Here's how the part is built. I have some questions about the finished solid (model axes, mm). A direction names the side the tool comes from. Round coordinates to 2 decimals unless told otherwise and drop trailing zeros. Write each loop counter-clockwise with the first axis right and the second up, starting at its lowest first coordinate (ties: lowest second). Pieces come first, ordered by that corner, then holes. Notation, with made-up numbers: (-36.5, 71.25) - (-7.5, 71.25) arc R10 ccw to (-7.5, 85.25) - close; hole circle Ø6 at (67.25, -0.75). An arc over 180 degrees is marked (long way). Return JSON: item names as keys, results as strings. Group by question number.
Autodesk Inventor part; units mm, degrees
ref_plane "YZ Plane" through (0, 0, 0) normal (1, 0, 0) x (0, 1, 0)
ref_plane "XZ Plane" through (0, 0, 0) normal (0, 1, 0) x (-1, 0, 0)
ref_plane "XY Plane" through (0, 0, 0) normal (0, 0, 1) x (1, 0, 0)
sketch "Sketch1" plane through (0, 0, 0) normal (0, 0, 1) x (1, 0, 0)
  line L0 (0, 0) -> (111, 0)
  line L1 (111, 0) -> (111, 66)
  line L2 (111, 66) -> (0, 66)
  line L3 (0, 66) -> (0, 0)
  line L4 (2, 2) -> (109, 2)
  line L5 (109, 2) -> (109, 64)
  line L6 (109, 64) -> (2, 64)
  line L7 (2, 64) -> (2, 2)
  line L8 (2, 64) -> (107, 64)
  line L9 (107, 64) -> (107, 2)
  line L10 (107, 2) -> (2, 2)
  line L11 (2, 2) -> (2, 64)
  line L12 (2, 64) -> (0, 64)
  line L13 (0, 64) -> (0, 2)
  line L14 (0, 2) -> (2, 2)
  line L15 (2, 2) -> (2, 64)
  line L16 (2, 64) -> (107, 64)
  line L17 (107, 64) -> (107, 62)
  line L18 (107, 62) -> (2, 62)
  line L19 (2, 62) -> (2, 64)
  line L20 (2, 2) -> (107, 2)
  line L21 (107, 2) -> (107, 4)
  line L22 (107, 4) -> (2, 4)
  line L23 (2, 4) -> (2, 2)
  point P0 (2, 64)
  point P1 (2, 2)
  point P2 (107, 2)
  point P3 (2, 4)
  point P4 (2, 62)
  dimension "d0" = 111
  dimension "d1" = 66
  dimension "d2" = 107
  dimension "d3" = 2
  dimension "d4" = 2
  dimension "d5" = 62
  dimension "d6" = 105
  dimension "d8" = 0
  dimension "d9" = 0
  dimension "d10" = 0
  dimension "d56" = 105
  dimension "d57" = 2
  dimension "d58" = 105
  dimension "d59" = 2
extrude "Extrusion1" add sketch "Sketch1" against normal blind 2
extrude "Extrusion2" add sketch "Sketch1" along normal blind 5 contours L9 L6 L5 L4
extrude "Extrusion3" add sketch "Sketch1" along normal blind 20 contours L3 L12 L7 L14
sketch "Sketch2" plane through (0, 0, 0) normal (0, 0, 1) x (1, 0, 0)
  line L0 (9, 58) -> (59, 58)
  line L1 (59, 58) -> (59, 8)
  line L2 (59, 8) -> (9, 8)
  line L3 (9, 8) -> (9, 58)
  line L4 (0, 64) -> (0, 2)
  line L5 (2, 64) -> (107, 64)
  line L6 (12.45, 54.55) -> (55.65, 54.55)
  line L7 (55.65, 54.55) -> (55.65, 11.35)
  line L8 (55.65, 11.35) -> (12.45, 11.35)
  line L9 (12.45, 11.35) -> (12.45, 54.55)
  circle A0 centre (12.45, 54.55) radius 1.55
  circle A1 centre (55.65, 54.55) radius 1.55
  circle A2 centre (12.45, 11.35) radius 1.55
  circle A3 centre (55.65, 11.35) radius 1.55
  circle A4 centre (12.45, 54.55) radius 3.5
  circle A5 centre (55.65, 54.55) radius 3.5
  circle A6 centre (55.65, 11.35) radius 3.5
  circle A7 centre (12.45, 11.35) radius 3.5
  line L10 (15.95, 18) -> (35.95, 18)
  line L11 (35.95, 18) -> (35.95, 8)
  line L12 (35.95, 8) -> (15.95, 8)
  line L13 (15.95, 8) -> (15.95, 18)
  line L14 (12.45, 54.55) -> (55.65, 11.35)
  line L15 (55.65, 54.55) -> (12.45, 11.35)
  line L16 (24.05, 22.95) -> (44.05, 22.95)
  line L17 (44.05, 22.95) -> (44.05, 42.95)
  line L18 (44.05, 42.95) -> (24.05, 42.95)
  line L19 (24.05, 42.95) -> (24.05, 22.95)
  line L20 (24.05, 22.95) -> (44.05, 42.95) construction
  line L21 (44.05, 22.95) -> (24.05, 42.95) construction
  line L22 (15.95, 58) -> (35.95, 58)
  line L23 (35.95, 58) -> (35.95, 48)
  line L24 (35.95, 48) -> (15.95, 48)
  line L25 (15.95, 48) -> (15.95, 58)
  point P0 (0, 0)
  point P1 (13.0395, 58)
  point P2 (11.8605, 58)
  point P3 (9, 55.1395)
  point P4 (9, 53.9605)
  point P5 (9, 11.9395)
  point P6 (9, 10.7605)
  point P7 (11.4363, 8)
  point P8 (13.4637, 8)
  point P9 (54.6363, 8)
  point P10 (56.6637, 8)
  point P11 (59, 10.3363)
  point P12 (59, 12.3637)
  point P13 (59, 53.5363)
  point P14 (59, 55.5637)
  point P15 (56.2395, 58)
  point P16 (55.0605, 58)
  point P17 (34.05, 32.95)
  dimension "d19" = 50
  dimension "d20" = 50
  dimension "d21" = 9
  dimension "d22" = 6
  dimension "d23" = 43.2
  dimension "d24" = 43.2
  dimension "d25" = 3.45
  dimension "d26" = 3.45
  dimension "d27" = 3.1
  dimension "d28" = 3.1
  dimension "d29" = 3.1
  dimension "d30" = 3.1
  dimension "d31" = 7
  dimension "d32" = 7
  dimension "d33" = 7
  dimension "d34" = 7
  dimension "d47" = 20
  dimension "d48" = 0
  dimension "d49" = 10
  dimension "d50" = 20
  dimension "d51" = 20
  dimension "d65" = 20
  dimension "d66" = 10
  dimension "d67" = 0
extrude "Extrusion5" add sketch "Sketch2" along normal blind 12 contours A4 L6 A0 L9 L3 L0 | L0 A4 | A4 L14 A0 L6 | A5 L0 | L0 A5 L1 L7 A1 L6 | A4 L9 A0 L14 | L6 A1 L15 A5 | L3 A4 | A5 L1 | L15 A1 L7 A5 | A7 L15 A2 L9 | L9 A2 L8 A7 L2 L3 | L3 A7 | A7 L8 A2 L15 | A6 L1 | L1 A6 L2 L8 A3 L7 | L7 A3 L14 A6 | L14 A3 L8 A6 | L2 A7 | A6 L2
chamfer "Chamfer1" distance 2 angle 45 4 edges at (55.5, 66, -2) (0, 33, -2) (55.5, 0, -2) (111, 33, -2)
sketch "Sketch3" plane through (0, 2, 20) normal (-1, 0, 0) x (0, 0, 1)
  line L0 (-20, 62) -> (0, 62)
  line L1 (-20, 62) -> (-20, 0)
  line L2 (0, 62) -> (-20, 0)
  line L3 (0, 62) -> (0, 0)
  line L4 (0, 0) -> (-20, 62)
  line L5 (-2, 51) -> (-18, 51)
  line L6 (-18, 51) -> (-18, 11)
  line L7 (-18, 11) -> (-2, 11)
  line L8 (-2, 11) -> (-2, 51)
  line L9 (-2, 51) -> (-18, 11) construction
  line L10 (-18, 51) -> (-2, 11) construction
  point P0 (-20, -2)
  point P1 (-15, 62)
  point P2 (-10, 31)
  dimension "d43" = 16
  dimension "d44" = 40
extrude "Extrusion6" cut sketch "Sketch3" along normal mid plane 10 contours L5 L2 L4 | L4 L2 L7 L6 L5 | L5 L8 L7 L4 L2 | L2 L4 L7
extrude "Extrusion7" cut sketch "Sketch2" against normal blind 10 contours L18 L15 L14 | L14 L15 L19 | L17 L14 L15 | L14 L16 L15
extrude "Extrusion9" add sketch "Sketch1" along normal blind 5 contours L7 L22 L9 L4 | L6 L9 L18 L7
chamfer "Chamfer3" distance 2 angle 45 2 edges at (0, 2, 10) (0, 64, 10)
extrude "Extrusion10" cut sketch "Sketch2" along normal mid plane 10 contours L0 L23 L6 L25 | L6 L23 L24 L14 L25 | L14 L24 L25
equation "\"d0\" = capLength"
equation "\"d1\" = capWidth"
equation "\"d2\" = capLength - 2 * wallWidth"
equation "\"d3\" = wallWidth"
equation "\"d4\" = wallWidth"
equation "\"d5\" = capWidth - 2 * wallWidth"
equation "\"d6\" = capLength - 3 * wallWidth"
equation "\"d56\" = capLength - 3 * wallWidth"
equation "\"d57\" = wallWidth"
equation "\"d58\" = capLength - 3 * wallWidth"
equation "\"d59\" = wallWidth"
equation "\"d11\" = wallWidth"
equation "\"d13\" = wallsHeight"
equation "\"d15\" = height"
equation "\"d19\" = PCBWidth"
equation "\"d20\" = PCBWidth"
equation "\"d21\" = connectorsLength"
equation "\"d22\" = -0.5 * PCBWidth + 0.5 * capWidth - wallWidth"
equation "\"d23\" = widthBetweenHoles"
equation "\"d24\" = widthBetweenHoles"
equation "\"d25\" = holesDistance"
equation "\"d26\" = holesDistance"
equation "\"d27\" = dHoles"
equation "\"d28\" = dHoles"
equation "\"d29\" = dHoles"
equation "\"d30\" = dHoles"
equation "\"d31\" = dBonks"
equation "\"d32\" = dBonks"
equation "\"d33\" = dBonks"
equation "\"d34\" = dBonks"
equation "\"d47\" = cutoutLength"
equation "\"d49\" = cutoutWidth"
equation "\"d50\" = switchersWidth"
equation "\"d51\" = switchersWidth"
equation "\"d65\" = cutoutLength"
equation "\"d66\" = cutoutWidth"
equation "\"d43\" = hWindow"
equation "\"d44\" = wWindow"
equation "\"d60\" = wallsHeight"
equation "\"capWidth\" = 66"
equation "\"capLength\" = 111"
equation "\"wallWidth\" = 2"
equation "\"wallsHeight\" = 5"
equation "\"height\" = 20"
equation "\"dHoles\" = 3.1"
equation "\"dBonks\" = 7"
equation "\"PCBWidth\" = 50"
equation "\"connectorsLength\" = 9"
equation "\"widthBetweenHoles\" = 43.2"
equation "\"holesDistance\" = 3.45"
equation "\"hWindowCenter\" = 8"
equation "\"hWindow\" = 16"
equation "\"wWindow\" = 40"
equation "\"cutoutLength\" = 20"
equation "\"cutoutWidth\" = 10"
equation "\"switchersWidth\" = 20"
properties part number "Cap"
1) Imagine slicing it at D-D (z = 16.75). Please give me the cut outline in (x, y), plus the area to 3 significant figures.
2) I need wall thicknesses on line 1 along Y through (x, z) = (12.45, 6.75); line 2 along X through (y, z) = (11.35, 7.25); line 3 along Y through (x, z) = (8, 3.5). Which ranges of each line are inside material? Lowest first, please.
3) If we mould it in two halves opening along X, with no side actions, what happens to faces 4 (the flat face through (107, 33, 2)), 5 (the flat face through (1, 33, 2)), 6 (the flat face through (110, 33, -1)), 7 (the cylindrical face through (54.1, 54.5, 5.9))? For each: released by +X, released by -X, zero draft, split by the parting line, or undercut.
4) For faces 1 (the flat face through (14, 10.6, 12)), 2 (the flat face through (55, 2, 2)), 3 (the flat face through (24.05, 33, -1)), which set-ups out of +Z, -Z, +X, -X, +Y, -Y let a thin tool reach every point of the face, with its end or its side?
5) Will these pins go through, and if not, where does the flat tip stop? pin 1 Ø4 at (y, z) = (16, 11) entering from +X; pin 2 Ø1.6 at (x, z) = (38, -1.5) entering from +Y; pin 3 Ø0.6 at (x, z) = (1.5, 9.5) entering from +Y; pin 4 Ø4 at (x, z) = (72, 1.5) entering from +Y.
6) Imagine slicing it at A-A (z = 3.5). Give the number of separate pieces and of enclosed holes in the cut face, plus the area to 3 significant figures.
Results found:
{
 "1": {"outline": "(0, 4) - (2, 2) - (2, 13) - (0, 13) - close; (0, 53) - (2, 53) - (2, 64) - (0, 62) - close", "area": "40.0 mm²"},
 "2": {"line 1": "y = 7.85 to 9.8, 12.9 to 14.85, 51.05 to 53, 56.1 to 58.05", "line 2": "x = 0 to 2, 8.95 to 10.9, 14 to 15.95, 52.15 to 54.1, 57.2 to 59.15", "line 3": "y = 2 to 4, 62 to 64"},
 "3": {"face 4": "undercut", "face 5": "zero draft", "face 6": "released by +X", "face 7": "undercut"},
 "4": {"face 1": "+Z, +X, +Y, -Y", "face 2": "+Z, +X, -X, -Y", "face 3": "+Z, -Z"},
 "5": {"pin 1": "stops at x = 57.94", "pin 2": "stops at y = 65.3", "pin 3": "stops at y = 63.8", "pin 4": "stops at y = 66"},
 "6": {"separate pieces": "5", "enclosed holes": "4", "area": "708 mm²"}
}
